Work out the finished part from the listing and answer in its coordinate system (mm). A direction names the side the tool comes from. Give positions to 0.01 mm unless a question says otherwise; leave off trailing zeros. Order: outer loops, then holes, each group sorted by start corner. A loop starts at its lowest first (then second) coordinate and runs counter-clockwise, first axis right, second up. Notation, with made-up numbers: M 41,76 L 57,76 A10 cw 57,93 Z; hole C 60.25,18.25 d7. An arc over 180 degrees is marked long. One line per item, written item: value.
from build123d import *

# Parameters (mm, degrees)
F1_DEPTH  = 6.35
F3_SIZE   = 3.175
F5_W      = 6.35
F5_H      = 6.35
F6_DEPTH  = 25.4
F2_R      = 15.875
F7_DEPTH  = 25.4
F8_W      = 10.16
F8_H      = 10.16
F8_W_2    = 6.35
F8_H_2    = 6.35
F9_DEPTH  = 5.08
F10_W     = 10.16
F10_H     = 10.16
F10_W_2   = 6.35
F10_H_2   = 6.35
F11_DEPTH = 5.08
F12_W     = 10.16
F12_H     = 10.16
F12_W_2   = 6.35
F12_H_2   = 6.35
F13_DEPTH = 5.08
F14_W     = 10.16
F14_H     = 10.16
F14_W_2   = 6.35
F14_H_2   = 6.35
F15_DEPTH = 5.08
F4_R      = 3.175
F16_DEPTH = 25.4


# Not quite as in the source:
# - a feature names something its author has since deleted; it is built from what else it names


with BuildPart() as f1:
    # F0 (on Front) → F1 (new body)
    with BuildSketch(Plane.XZ):
        Polygon((139.7, 0), (0, 0), (0, -139.7), (38.1, -139.7), (38.1, -114.3), (63.5, -114.3), (63.5, -88.9), (88.9, -88.9), (88.9, -63.5), (114.3, -63.5), (114.3, -38.1), (139.7, -38.1), align=None)
    extrude(amount=F1_DEPTH)

    # F3
    f3_edges = [f1.edges().sort_by_distance(p)[0] for p in [
        (69.85, -6.35, 0),
        (0, -6.35, -69.85),
        (19.05, -6.35, -139.7),
        (38.1, -6.35, -127),
        (50.8, -6.35, -114.3),
        (63.5, -6.35, -101.6),
        (76.2, -6.35, -88.9),
        (88.9, -6.35, -76.2),
        (101.6, -6.35, -63.5),
        (114.3, -6.35, -50.8),
        (127, -6.35, -38.1),
        (139.7, -6.35, -19.05),
    ]]
    chamfer(f3_edges, length=F3_SIZE)

    # F5 (on face) → F6 (join)
    with BuildSketch(Plane(origin=(0, 0, 0), x_dir=(-1, 0, 0), z_dir=(0, 1, 0))):
        with Locations((-3.175, -3.175)):
            Rectangle(F5_W, F5_H)
        with Locations((-3.175, -136.525)):
            Rectangle(F5_W, F5_H)
        with Locations((-85.725, -85.725)):
            Rectangle(F5_W, F5_H)
        with Locations((-136.525, -3.175)):
            Rectangle(F5_W, F5_H)
    extrude(amount=F6_DEPTH)

    # F2 (on face) → F7 (cut)
    with BuildSketch(Plane.XZ.offset(6.35)):
        with BuildLine():
            ThreePointArc((117.475, -22.86), (90.3746798487, -11.6346798487), (101.6, -38.735))
            Line((101.6, -38.735), (101.6, -22.86))
            Line((101.6, -22.86), (117.475, -22.86))
        make_face()
        with BuildLine():
            Line((101.6, -22.86), (101.6, -38.735))
            ThreePointArc((101.6, -38.735), (112.8253201513, -34.0853201513), (117.475, -22.86))
            Line((117.475, -22.86), (101.6, -22.86))
        make_face()
        with BuildLine():
            ThreePointArc((82.3243596973, -66.4493596973), (51.7827721187, -60.3742602085), (77.6746798487, -77.6746798487))
            ThreePointArc((77.6746798487, -77.6746798487), (81.1159472759, -72.5244591861), (82.3243596973, -66.4493596973))
        make_face()
        with Locations((22.86, -101.6)):
            Circle(F2_R)
        with BuildLine():
            ThreePointArc((38.3256403027, -22.4506403027), (28.5257397915, -7.7840527241), (11.2253201513, -11.2253201513))
            ThreePointArc((11.2253201513, -11.2253201513), (16.3755408139, -37.1172278813), (38.3256403027, -22.4506403027))
        make_face()
    extrude(amount=-F7_DEPTH, mode=Mode.SUBTRACT)

    # F8 (on face) → F9 (join)
    with BuildSketch(Plane(origin=(0, 25.4, 0), x_dir=(-1, 0, 0), z_dir=(0, 1, 0))):
        with Locations((-3.175, -3.175)):
            Rectangle(F8_W, F8_H)
        with Locations((-3.175, -3.175)):
            Rectangle(F8_W_2, F8_H_2, mode=Mode.SUBTRACT)
        with Locations((-3.175, -3.175)):
            Rectangle(F8_W_2, F8_H_2)
    extrude(amount=F9_DEPTH)

    # F10 (on face) → F11 (join)
    with BuildSketch(Plane(origin=(0, 25.4, 0), x_dir=(-1, 0, 0), z_dir=(0, 1, 0))):
        with Locations((-136.525, -3.175)):
            Rectangle(F10_W, F10_H)
        with Locations((-136.525, -3.175)):
            Rectangle(F10_W_2, F10_H_2, mode=Mode.SUBTRACT)
        with Locations((-136.525, -3.175)):
            Rectangle(F10_W_2, F10_H_2)
    extrude(amount=F11_DEPTH)

    # F12 (on face) → F13 (join)
    with BuildSketch(Plane(origin=(0, 25.4, 0), x_dir=(-1, 0, 0), z_dir=(0, 1, 0))):
        with Locations((-85.725, -85.725)):
            Rectangle(F12_W, F12_H)
        with Locations((-85.725, -85.725)):
            Rectangle(F12_W_2, F12_H_2, mode=Mode.SUBTRACT)
        with Locations((-85.725, -85.725)):
            Rectangle(F12_W_2, F12_H_2)
    extrude(amount=F13_DEPTH)

    # F14 (on face) → F15 (join)
    with BuildSketch(Plane(origin=(0, 25.4, 0), x_dir=(-1, 0, 0), z_dir=(0, 1, 0))):
        with Locations((-3.175, -136.525)):
            Rectangle(F14_W, F14_H)
        with Locations((-3.175, -136.525)):
            Rectangle(F14_W_2, F14_H_2, mode=Mode.SUBTRACT)
        with Locations((-3.175, -136.525)):
            Rectangle(F14_W_2, F14_H_2)
    extrude(amount=F15_DEPTH)

    # F4 (on face) → F16 (cut)
    with BuildSketch(Plane.XZ.offset(6.35)):
        with Locations((63.5, -28.575)):
            Circle(F4_R)
        with Locations((28.575, -63.5)):
            Circle(F4_R)
    extrude(amount=-F16_DEPTH, mode=Mode.SUBTRACT)


solid = f1.part
(1) Which of the six approach directions +Z, -Z, +X, -X, +Y, -Y give full straight-line access (tool end or side, diameter ignored) to faces 4 (the flat face through (127, -2, -38.1)), 5 (the flat face through (86, 28, -80.645)), 6 (the flat face through (74.412, -4.785, -87.29))?
Findings:
face 4: -Z, +X, +Y, -Y
face 5: +Z, +X, -X, +Y
face 6: -Z, +X, -Y
(2) Section C-C, the plane x = 95.5 is taken. Give the vertices of the cut face in (y, z) (3 decimals), then the cut area to 3 significant figures.
Findings:
outline: M -6.35,-60.325 L -3.175,-63.5 L 0,-63.5 L 0,-37.516 L -6.35,-37.516 Z; M -6.35,-8.204 L 0,-8.204 L 0,0 L -3.175,0 L -6.35,-3.175 Z
area: 207 mm^2
(3) Find the intervals of material crossed by probe 1 along X at (y, z) = (-1.75, -22.86) (3 decimals); probe 2 along X at (y, z) = (-4, -63) (3 decimals); probe 3 along Z at (x, y) = (22.86, -4.5) (3 decimals), in increasing order. Write a range as from..to.
Findings:
probe 1: x = 0..6.581, 38.32..85.725, 117.475..139.7
probe 2: x = 0.825..25.44, 31.71..50.954, 81.945..88.075
probe 3: z = -138.375..-117.475, -85.725..-38.32, -6.581..-1.325
(4) Determine the mould class of faces 1 (the flat face through (133.35, 13, -3)), 2 (the flat face through (137, 28, 1.905)), 3 (the flat face through (114.3, -2, -51)) for opening direction X: pulls with the +X half, pulls with the -X half, needs draft (parallel to the pull), parting line crosses it, or undercut.
Findings:
face 1: undercut
face 2: needs draft
face 3: pulls with the +X half
(5) Section B-B, the plane z = -101.6 is taken. Give the vertices of the cut face in (x, y) (3 decimals), then the cut area to 3 significant figures.
Findings:
outline: M 0,-3.175 L 3.175,-6.35 L 6.985,-6.35 L 6.985,0 L 0,0 Z; M 38.735,-6.35 L 60.325,-6.35 L 63.5,-3.175 L 63.5,0 L 38.735,0 Z
area: 192 mm^2
(6) Section A-A, the plane y = 20.5 is taken. Give the vertices of the cut face in (x, z).
Findings:
outline: M 0,-139.7 L 6.35,-139.7 L 6.35,-133.35 L 0,-133.35 Z; M 0,-6.35 L 6.35,-6.35 L 6.35,0 L 0,0 Z; M 82.55,-88.9 L 88.9,-88.9 L 88.9,-82.55 L 82.55,-82.55 Z; M 133.35,-6.35 L 139.7,-6.35 L 139.7,0 L 133.35,0 Z
(7) Section D-D, the plane z = -42 is taken. Give the vertices of the cut face in (x, y) (3 decimals).
Findings:
outline: M 0,-3.175 L 3.175,-6.35 L 111.125,-6.35 L 114.3,-3.175 L 114.3,0 L 0,0 Z
(8) Given P1, Ø1.5, axis at y = 28.5, z = -87.5, coming from the -X side (3 decimals); P2, Ø12, axis at x = 67.5, z = -52, coming from the +Y side; P3, Ø5, axis at y = 13, z = -92.5, coming from the -X side; P4, Ø5, axis at x = 2, y = 10, coming from the +Z side, each flat-ended and moving along its own axis, determine where each tip first touches the part or whether it passes through.
Findings:
P1: stops at x = 80.645
P2: stops at y = 0
P3: passes through
P4: stops at z = 0
